Work out the finished part from the listing and answer in its coordinate system (mm). Coordinates: 2 decimals unless noted, no trailing zeros. Order: outer loops, then holes, each group sorted by start corner. A loop starts at its lowest first (then second) coordinate and runs counter-clockwise, first axis right, second up. Notation, with made-up numbers: (69, 72.5) -> (74, 72.5) arc R18 ccw to (74, 90.5) -> close; hole circle Ø3 at (-13, -11). An arc over 180 degrees is marked (long way). Write item = value, one per line. Start each with the question number.
Q1. The part is cut by section C-C, the plane x = 0. Determine the outline of the cut face in (y, z).
Q2. Straight lines are drawn through the part: L1, parallel to Y at x = 0, z = 1; L2, parallel to Y at x = 7, z = 2.05; L3, parallel to X at y = 96.5, z = 4.1. For each, find the intervals that lie inside material, in ascending order. Write a range as from..to.
Q3. A flat-ended cylindrical pin translates along its axis: pin 1 (6 mm diameter, centred on x = 24.75, y = 48.25, fed in from +Z). Find the tip coordinate at first contact, or state that the pin passes through.
Q4. The part is cut by section A-A, the plane y = 97.75. Determine the outline of the cut face in (x, z), plus the area to 3 significant figures.
Q5. The part is cut by section B-B, the plane z = 1.75. Count the separate pieces of the cut face and the enclosed holes in it, plus the area to 3 significant figures.
Q6. The part is cut by section D-D, the plane y = -20.5. Determine the outline of the cut face in (x, z).
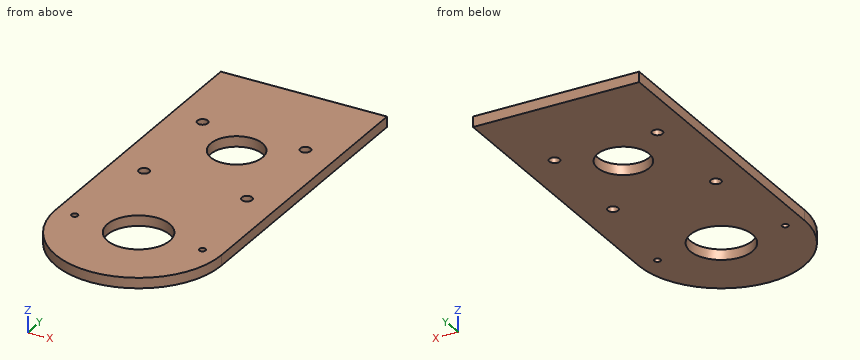
```python
from build123d import *

# Parameters (mm, degrees)
SKETCH1_R           = 15
BOSS_EXTRUDE1_DEPTH = 5
SKETCH2_R           = 2.5
SKETCH2_R_2         = 12.5
CUT_EXTRUDE1_DEPTH  = 146.688022843
SKETCH3_R           = 1.5
CUT_EXTRUDE2_DEPTH  = 10


with BuildPart() as part:
    # Sketch1 → Boss-Extrude1 (new body)
    with BuildSketch(Plane.XY):
        with BuildLine():
            Line((-40, 0), (-40, 140))
            Line((-40, 140), (40, 140))
            Line((40, 140), (40, 0))
            ThreePointArc((40, 0), (0, -40), (-40, 0))
        make_face()
        Circle(SKETCH1_R, mode=Mode.SUBTRACT)
    extrude(amount=BOSS_EXTRUDE1_DEPTH)

    # Sketch2 → Cut-Extrude1 (cut, through all)
    with BuildSketch(Plane(origin=(0, 0, 0), x_dir=(-1, 0, 0), z_dir=(0, 0, -1))):
        with Locations((-24.75, 97.75)):
            Circle(SKETCH2_R)
        with Locations((24.75, 97.75)):
            Circle(SKETCH2_R)
        with Locations((24.75, 48.25)):
            Circle(SKETCH2_R)
        with Locations((-24.75, 48.25)):
            Circle(SKETCH2_R)
        with Locations((0, 83)):
            Circle(SKETCH2_R_2)
    extrude(amount=-CUT_EXTRUDE1_DEPTH, mode=Mode.SUBTRACT)

    # Sketch3 → Cut-Extrude2 (cut)
    with BuildSketch(Plane(origin=(0, 0, 0), x_dir=(-1, 0, 0), z_dir=(0, 0, -1))):
        with Locations((-30.75, 0)):
            Circle(SKETCH3_R)
        with Locations((30.75, 0)):
            Circle(SKETCH3_R)
    extrude(amount=-CUT_EXTRUDE2_DEPTH, mode=Mode.SUBTRACT)


solid = part.part
```
Model answer:
q1.outline = (-40, 0) -> (-15, 0) -> (-15, 5) -> (-40, 5) -> close; (15, 0) -> (70.5, 0) -> (70.5, 5) -> (15, 5) -> close; (95.5, 0) -> (140, 0) -> (140, 5) -> (95.5, 5) -> close
q2.L1 = -40..-15, 15..70.5, 95.5..140
q2.L2 = -39.38..-13.27, 13.27..72.64, 93.36..140
q2.L3 = -40..-26.92, -22.58..22.58, 26.92..40
q3.pin_1 = 5
q4.outline = (-40, 0) -> (-27.25, 0) -> (-27.25, 5) -> (-40, 5) -> close; (-22.25, 0) -> (22.25, 0) -> (22.25, 5) -> (-22.25, 5) -> close; (27.25, 0) -> (40, 0) -> (40, 5) -> (27.25, 5) -> close
q4.area = 350 mm2
q5.separate_pieces = 1
q5.enclosed_holes = 8
q5.area = 12,400 mm2
q6.outline = (-34.35, 0) -> (34.35, 0) -> (34.35, 5) -> (-34.35, 5) -> close
